Verification items for this drawing (mm, ordinates from the low corner). Coordinates: 2 decimals unless noted, no trailing zeros. Order: outer loops, then holes, each group sorted by start corner. A loop starts at its lowest first (then second) coordinate and runs counter-clockwise, first axis right, second up.
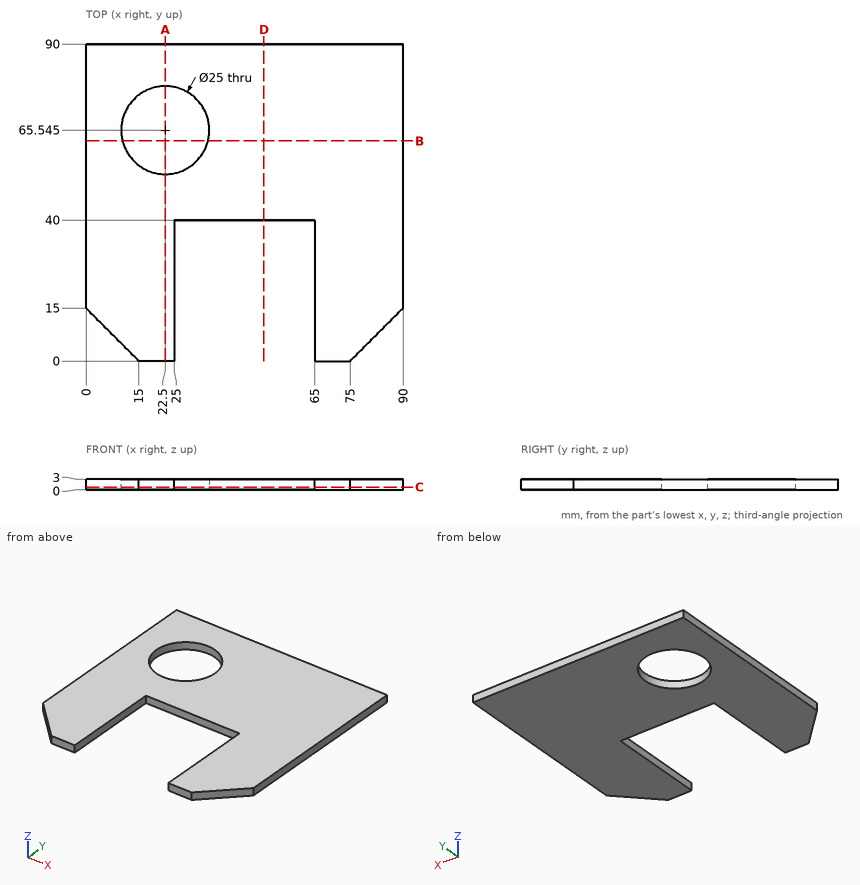
(1) Thickness scan on probe 1 along X at (y, z) = (22, 2.6); probe 2 along Y at (x, z) = (22.5, 0.75) (1 decimal); probe 3 along Y at (x, z) = (5, 1.8). Record the ranges inside material, lowest first.
Filled in:
probe 1: x = 0 to 25, 65 to 90
probe 2: y = 0 to 53, 78 to 90
probe 3: y = 10 to 90
(2) Cross-section at C-C (z = 0.7). Enter the section's corners in (x, y) (1 decimal).
Filled in:
outline: (0, 15) - (15, 0) - (25, 0) - (25, 40) - (65, 40) - (65, 0) - (75, 0) - (90, 15) - (90, 90) - (0, 90) - close; hole circle Ø25 at (22.5, 65.5)
(3) Go/stop test with a flat-tipped pin: P1, Ø0.9, axis at x = 49.5, z = 1.5, coming from the -Y side. Record where the tip stops, or that it passes through.
Filled in:
P1: stops at y = 40
(4) Cross-section at B-B (y = 62.5). Enter the section's corners in (x, z).
Filled in:
outline: (0, 0) - (10.38, 0) - (10.38, 3) - (0, 3) - close; (34.62, 0) - (90, 0) - (90, 3) - (34.62, 3) - close
(5) Cross-section at D-D (x = 50.5). Enter the section's corners in (y, z), and give its area (3 significant figures).
Filled in:
outline: (40, 0) - (90, 0) - (90, 3) - (40, 3) - close
area: 150 mm2
(6) Cross-section at A-A (x = 22.5). Enter the section's corners in (y, z) (1 decimal).
Filled in:
outline: (0, 0) - (53, 0) - (53, 3) - (0, 3) - close; (78, 0) - (90, 0) - (90, 3) - (78, 3) - close
